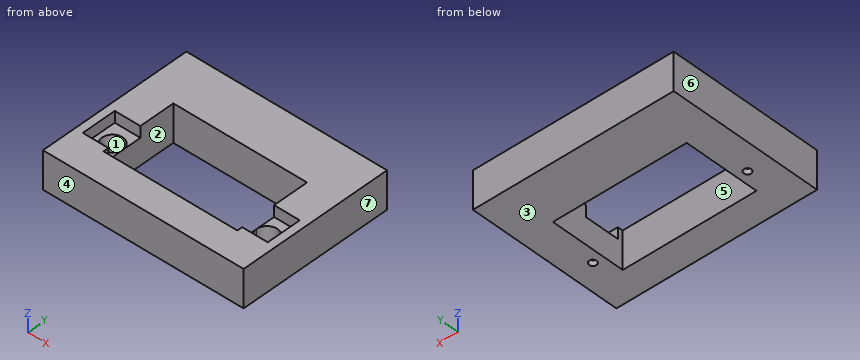
from build123d import *

# Parameters (mm, degrees)
BOX007_W        = 96
BOX007_H        = 74
BOX007_DEPTH    = 18
SKETCH047_R     = 1.75
POCKET015_DEPTH = 18.001
SKETCH048_W     = 64
SKETCH048_H     = 36
POCKET016_DEPTH = 18.001
SKETCH049_W     = 88.5
SKETCH049_H     = 16.5
POCKET017_DEPTH = 5.4
SKETCH050_R     = 5
POCKET018_DEPTH = 10


with BuildPart() as part:
    # Box007 → Box007 (new body)
    with BuildSketch(Plane(origin=(36, -80, 104), x_dir=(1, 0, 0), z_dir=(0, 0, 1))):
        with Locations((48, 37)):
            Rectangle(BOX007_W, BOX007_H)
    extrude(amount=BOX007_DEPTH)

    # Sketch047 → Pocket015 (cut, through all)
    with BuildSketch(Plane(origin=(36, -80, 122), x_dir=(1, 0, 0), z_dir=(0, 0, 1))):
        with Locations((11, 24)):
            Circle(SKETCH047_R)
        with Locations((85, 24)):
            Circle(SKETCH047_R)
    extrude(amount=-POCKET015_DEPTH, mode=Mode.SUBTRACT)

    # Sketch048 → Pocket016 (cut, through all)
    with BuildSketch(Plane(origin=(36, -80, 122), x_dir=(1, 0, 0), z_dir=(0, 0, 1))):
        with Locations((48, 32)):
            Rectangle(SKETCH048_W, SKETCH048_H)
    extrude(amount=-POCKET016_DEPTH, mode=Mode.SUBTRACT)

    # Sketch049 → Pocket017 (cut)
    with BuildSketch(Plane(origin=(36, -80, 122), x_dir=(1, 0, 0), z_dir=(0, 0, 1))):
        with Locations((48, 24.75)):
            Rectangle(SKETCH049_W, SKETCH049_H)
    extrude(amount=-POCKET017_DEPTH, mode=Mode.SUBTRACT)

    # Sketch050 → Pocket018 (cut)
    with BuildSketch(Plane(origin=(36, -80, 116.6), x_dir=(1, 0, 0), z_dir=(0, 0, 1))):
        with Locations((11, 24)):
            Circle(SKETCH050_R)
        with Locations((85, 24)):
            Circle(SKETCH050_R)
    extrude(amount=-POCKET018_DEPTH, mode=Mode.SUBTRACT)


solid = part.part
Part model, mm, in its own coordinate system. Face numbers are marked on the shaded views. A direction names the side the tool comes from. Give positions to 0.01 mm unless a question says otherwise; leave off trailing zeros. Loops run counter-clockwise (first coordinate to the right, second up) from the corner with the lowest first, then second, coordinate; pieces in that order, holes last.
(1) Pull direction X, two halves, no side cores. Call the marked faces 4, 5, 6 and 7: pulls with the +X half, pulls with the -X half, needs draft (parallel to the pull), parting line crosses it, or undercut.
Return value:
face 4: needs draft
face 5: undercut
face 6: pulls with the -X half
face 7: pulls with the +X half
(2) Band-saw the part on A-A (x = 121). Write the cut outline in (y, z).
Return value:
outline: (-80, 104) - (-57.75, 104) - (-57.75, 106.6) - (-61, 106.6) - (-61, 116.6) - (-63.5, 116.6) - (-63.5, 122) - (-80, 122) - close; (-54.25, 104) - (-6, 104) - (-6, 122) - (-47, 122) - (-47, 116.6) - (-51, 116.6) - (-51, 106.6) - (-54.25, 106.6) - close
(3) Band-saw the part on D-D (x = 80). Write the cut outline in (y, z).
Return value:
outline: (-80, 104) - (-66, 104) - (-66, 122) - (-80, 122) - close; (-30, 104) - (-6, 104) - (-6, 122) - (-30, 122) - close
(4) 3-axis set-ups, long thin cutter, end or side, ignore diameter. For the marked faces 1, 2 and 3: which of +Z, -Z, +X, -X, +Y, -Y reach the whole face in a straight line?
Return value:
face 1: +Z
face 2: +Z, -Z
face 3: -Z, +X, -X, +Y, -Y
(5) Drill centre lines: line 1 along Y through (x, z) = (71, 120.75); line 2 along Y through (x, z) = (120.5, 117.25); line 3 along X through (y, z) = (-50, 117.75). Where is each one in solid material? Low to high.
Return value:
line 1: y = -80 to -66, -30 to -6
line 2: y = -80 to -63.5, -47 to -6
line 3: x = 36 to 39.75, 128.25 to 132
(6) Pin check, flat tips, straight feed: pin 1 (3 mm diameter, centred on x = 121, y = -56, fed in from -Z); pin 2 (5 mm diameter, centred on x = 119.5, y = -56.5, fed in from +Z). Stop position of each tip, or through.
Return value:
pin 1: passes through
pin 2: stops at z = 106.6
(7) Band-saw the part on B-B (y = -34.5). Write the cut outline in (x, z).
Return value:
outline: (36, 104) - (52, 104) - (52, 122) - (36, 122) - close; (116, 104) - (132, 104) - (132, 122) - (116, 122) - close
